from build123d import *

# Parameters (mm, degrees)
SKETCH1_W           = 30
SKETCH1_H           = 41
SKETCH1_R           = 2.25
BOSS_EXTRUDE1_DEPTH = 12
SKETCH3_R           = 3.8
CUT_EXTRUDE2_DEPTH  = 7
FILLET1_R           = 2
SKETCH4_R           = 2.25
CUT_EXTRUDE3_DEPTH  = 53.201532625
CUT_EXTRUDE4_START  = -30
SKETCH5_R           = 3.75
CUT_EXTRUDE4_DEPTH  = 6


with BuildPart() as part:
    # Sketch1 → Boss-Extrude1 (new body)
    with BuildSketch(Plane(origin=(0, 0, 0), x_dir=(1, 0, 0), z_dir=(0, 1, 0))):
        with Locations((-15, 20.5)):
            Rectangle(SKETCH1_W, SKETCH1_H)
        with Locations(Location((-5, 6, 0), (0, 0, 270))):
            Circle(SKETCH1_R, mode=Mode.SUBTRACT)
        with Locations(Location((-5, 26, 0), (0, 0, 270))):
            Circle(SKETCH1_R, mode=Mode.SUBTRACT)
    extrude(amount=BOSS_EXTRUDE1_DEPTH)

    # Sketch3 → Cut-Extrude2 (cut)
    with BuildSketch(Plane(origin=(0, 12, 0), x_dir=(1, 0, 0), z_dir=(0, 1, 0))):
        with Locations(Location((-5, 26, 0), (0, 0, 270))):
            Circle(SKETCH3_R)
        with Locations(Location((-5, 6, 0), (0, 0, 270))):
            Circle(SKETCH3_R)
    extrude(amount=-CUT_EXTRUDE2_DEPTH, mode=Mode.SUBTRACT)

    # Fillet1
    # the kernel refuses this fillet: 2 mm, written as the material it takes off along each edge
    with BuildSketch(Plane(origin=(-28, 10, -2), x_dir=(-1, 0, 0), z_dir=(0, 0, 1))) as fillet1_piece_1_section:
        Polygon((0, 0), (FILLET1_R, 0), (FILLET1_R, -FILLET1_R), (0, -FILLET1_R), align=None)
    fillet1_piece_1 = extrude(amount=FILLET1_R, mode=Mode.PRIVATE)
    fillet1_piece_1 = fillet1_piece_1 - Plane(origin=(-28, 10, -2), x_dir=(0.7071067811865475, -0.7071067811865475, 0), z_dir=(0, 0, 1)) * Sphere(FILLET1_R, mode=Mode.PRIVATE)
    add(fillet1_piece_1, mode=Mode.SUBTRACT)
    with BuildSketch(Plane(origin=(-28, 10, -39), x_dir=(0, 1, 0), z_dir=(-1, 0, 0))) as fillet1_piece_2_section:
        Polygon((0, 0), (FILLET1_R, 0), (FILLET1_R, FILLET1_R), (0, FILLET1_R), align=None)
    fillet1_piece_2 = extrude(amount=FILLET1_R, mode=Mode.PRIVATE)
    fillet1_piece_2 = fillet1_piece_2 - Plane(origin=(-28, 10, -39), x_dir=(0, -0.7071067811865475, 0.7071067811865475), z_dir=(-1, 0, 0)) * Sphere(FILLET1_R, mode=Mode.PRIVATE)
    add(fillet1_piece_2, mode=Mode.SUBTRACT)
    with BuildSketch(Plane(origin=(-2, 10, -2), x_dir=(1, 0, 0), z_dir=(0, 0, 1))) as fillet1_piece_3_section:
        Polygon((0, 0), (FILLET1_R, 0), (FILLET1_R, FILLET1_R), (0, FILLET1_R), align=None)
    fillet1_piece_3 = extrude(amount=FILLET1_R, mode=Mode.PRIVATE)
    fillet1_piece_3 = fillet1_piece_3 - Plane(origin=(-2, 10, -2), x_dir=(-0.7071067811865475, -0.7071067811865475, 0), z_dir=(0, 0, 1)) * Sphere(FILLET1_R, mode=Mode.PRIVATE)
    add(fillet1_piece_3, mode=Mode.SUBTRACT)
    with BuildSketch(Plane(origin=(-2, 10, -39), x_dir=(0, 1, 0), z_dir=(1, 0, 0))) as fillet1_piece_4_section:
        Polygon((0, 0), (FILLET1_R, 0), (FILLET1_R, -FILLET1_R), (0, -FILLET1_R), align=None)
    fillet1_piece_4 = extrude(amount=FILLET1_R, mode=Mode.PRIVATE)
    fillet1_piece_4 = fillet1_piece_4 - Plane(origin=(-2, 10, -39), x_dir=(0, -0.7071067811865475, 0.7071067811865475), z_dir=(1, 0, 0)) * Sphere(FILLET1_R, mode=Mode.PRIVATE)
    add(fillet1_piece_4, mode=Mode.SUBTRACT)
    with BuildSketch(Plane(origin=(-2, 2, -2), x_dir=(1, 0, 0), z_dir=(0, 0, 1))) as fillet1_piece_5_section:
        Polygon((0, 0), (FILLET1_R, 0), (FILLET1_R, -FILLET1_R), (0, -FILLET1_R), align=None)
    fillet1_piece_5 = extrude(amount=FILLET1_R, mode=Mode.PRIVATE)
    fillet1_piece_5 = fillet1_piece_5 - Plane(origin=(-2, 2, -2), x_dir=(-0.7071067811865475, 0.7071067811865475, 0), z_dir=(0, 0, 1)) * Sphere(FILLET1_R, mode=Mode.PRIVATE)
    add(fillet1_piece_5, mode=Mode.SUBTRACT)
    with BuildSketch(Plane(origin=(-28, 2, -2), x_dir=(-1, 0, 0), z_dir=(0, 0, 1))) as fillet1_piece_6_section:
        Polygon((0, 0), (FILLET1_R, 0), (FILLET1_R, FILLET1_R), (0, FILLET1_R), align=None)
    fillet1_piece_6 = extrude(amount=FILLET1_R, mode=Mode.PRIVATE)
    fillet1_piece_6 = fillet1_piece_6 - Plane(origin=(-28, 2, -2), x_dir=(0.7071067811865475, 0.7071067811865475, 0), z_dir=(0, 0, 1)) * Sphere(FILLET1_R, mode=Mode.PRIVATE)
    add(fillet1_piece_6, mode=Mode.SUBTRACT)
    with BuildSketch(Plane(origin=(-28, 2, -39), x_dir=(0, -1, 0), z_dir=(-1, 0, 0))) as fillet1_piece_7_section:
        Polygon((0, 0), (FILLET1_R, 0), (FILLET1_R, -FILLET1_R), (0, -FILLET1_R), align=None)
    fillet1_piece_7 = extrude(amount=FILLET1_R, mode=Mode.PRIVATE)
    fillet1_piece_7 = fillet1_piece_7 - Plane(origin=(-28, 2, -39), x_dir=(0, 0.7071067811865475, 0.7071067811865475), z_dir=(-1, 0, 0)) * Sphere(FILLET1_R, mode=Mode.PRIVATE)
    add(fillet1_piece_7, mode=Mode.SUBTRACT)
    with BuildSketch(Plane(origin=(-2, 2, -39), x_dir=(0, -1, 0), z_dir=(1, 0, 0))) as fillet1_piece_8_section:
        Polygon((0, 0), (FILLET1_R, 0), (FILLET1_R, FILLET1_R), (0, FILLET1_R), align=None)
    fillet1_piece_8 = extrude(amount=FILLET1_R, mode=Mode.PRIVATE)
    fillet1_piece_8 = fillet1_piece_8 - Plane(origin=(-2, 2, -39), x_dir=(0, 0.7071067811865475, 0.7071067811865475), z_dir=(1, 0, 0)) * Sphere(FILLET1_R, mode=Mode.PRIVATE)
    add(fillet1_piece_8, mode=Mode.SUBTRACT)
    with BuildSketch(Plane(origin=(-30, 12, -2), x_dir=(0, -1, 0), z_dir=(0, 0, -1)), Plane(origin=(0, 12, -39), x_dir=(0, -1, 0), z_dir=(0, 0, 1))) as fillet1_piece_9:
        with BuildLine():
            CenterArc((FILLET1_R, -FILLET1_R), FILLET1_R, 90, 90)
            Line((0, -FILLET1_R), (0, 0))
            Line((0, 0), (FILLET1_R, 0))
        make_face()
    extrude(amount=37, mode=Mode.SUBTRACT)
    with BuildSketch(Plane(origin=(-2, 12, 0), x_dir=(0, -1, 0), z_dir=(-1, 0, 0)), Plane(origin=(-28, 0, -41), x_dir=(0, 0, 1), z_dir=(1, 0, 0))) as fillet1_piece_10:
        with BuildLine():
            CenterArc((FILLET1_R, -FILLET1_R), FILLET1_R, 90, 90)
            Line((0, -FILLET1_R), (0, 0))
            Line((0, 0), (FILLET1_R, 0))
        make_face()
    extrude(amount=26, mode=Mode.SUBTRACT)
    with BuildSketch(Plane(origin=(-2, 0, 0), x_dir=(0, 1, 0), z_dir=(-1, 0, 0)), Plane(origin=(-28, 12, -41), x_dir=(0, 0, 1), z_dir=(1, 0, 0))) as fillet1_piece_11:
        with BuildLine():
            CenterArc((FILLET1_R, FILLET1_R), FILLET1_R, 180, 90)
            Line((0, FILLET1_R), (0, 0))
            Line((0, 0), (FILLET1_R, 0))
        make_face()
    extrude(amount=26, mode=Mode.SUBTRACT)
    with BuildSketch(Plane(origin=(-30, 0, -2), x_dir=(0, 1, 0), z_dir=(0, 0, -1)), Plane(origin=(0, 0, -39), x_dir=(0, 1, 0), z_dir=(0, 0, 1))) as fillet1_piece_12:
        with BuildLine():
            CenterArc((FILLET1_R, FILLET1_R), FILLET1_R, 180, 90)
            Line((0, FILLET1_R), (0, 0))
            Line((0, 0), (FILLET1_R, 0))
        make_face()
    extrude(amount=37, mode=Mode.SUBTRACT)
    with BuildSketch(Plane(origin=(0, 2, 0), x_dir=(-1, 0, 0), z_dir=(0, 1, 0)), Plane(origin=(0, 2, -41), x_dir=(0, 0, 1), z_dir=(0, 1, 0))) as fillet1_piece_13:
        with BuildLine():
            CenterArc((FILLET1_R, -FILLET1_R), FILLET1_R, 90, 90)
            Line((0, -FILLET1_R), (0, 0))
            Line((0, 0), (FILLET1_R, 0))
        make_face()
    extrude(amount=8, mode=Mode.SUBTRACT)
    with BuildSketch(Plane(origin=(-30, 2, 0), x_dir=(1, 0, 0), z_dir=(0, 1, 0)), Plane(origin=(-30, 2, -41), x_dir=(0, 0, 1), z_dir=(0, 1, 0))) as fillet1_piece_14:
        with BuildLine():
            CenterArc((FILLET1_R, FILLET1_R), FILLET1_R, 180, 90)
            Line((0, FILLET1_R), (0, 0))
            Line((0, 0), (FILLET1_R, 0))
        make_face()
    extrude(amount=8, mode=Mode.SUBTRACT)

    # Sketch4 → Cut-Extrude3 (cut, through all)
    with BuildSketch(Plane.ZY.offset(30)):
        with Locations((-34, 5.5)):
            Circle(SKETCH4_R)
        with Locations((-18, 5.5)):
            Circle(SKETCH4_R)
    extrude(amount=-CUT_EXTRUDE3_DEPTH, mode=Mode.SUBTRACT)

    # Sketch5 → Cut-Extrude4 (cut)
    with BuildSketch(Plane.ZY.offset(30).offset(CUT_EXTRUDE4_START)):
        with Locations(Location((-34, 5.5, 0), (0, 0, 248.960530219))):
            Circle(SKETCH5_R)
        with Locations(Location((-18, 5.5, 0), (0, 0, 248.960530219))):
            Circle(SKETCH5_R)
    extrude(amount=CUT_EXTRUDE4_DEPTH, mode=Mode.SUBTRACT)


solid = part.part
Check sheet for the modelled part. Datum: model origin and axes. Units: mm. A direction names the side the tool comes from. Round coordinates to 2 decimals unless told otherwise and drop trailing zeros. Write each loop counter-clockwise with the first axis right and the second up, starting at its lowest first coordinate (ties: lowest second). Pieces come first, ordered by that corner, then holes. Notation, with made-up numbers: (36, 62.25) -> (90, 62.25) arc R30 ccw to (90, 90.25) -> close; hole circle Ø7 at (40.5, 28). An arc over 180 degrees is marked (long way). Answer as CSV lines item,"result". Start each with the question number.
1) Tool access check on faces 5 (the cylindrical face through (-0.57, 11.4, -20.76)), 6 (the cylindrical face through (-6.46, 8.55, -2.49)), 7 (the cylindrical face through (-2.958, 1.757, -18.233)). Record the directions out of +Z, -Z, +X, -X, +Y, -Y that give a thin tool (end or side, any length) a straight path to the whole face; none if there is none.
2) Section check B-B on x = -5.5. Enter the section's corners in (y, z).
3) Go/stop test with flat-tipped pins: P1, Ø4, axis at y = 5.5, z = -33.5, coming from the +X side; P2, Ø1, axis at x = -7, z = -10, coming from the -Y side; P3, Ø7, axis at x = -5, z = -6, coming from the +Y side; P4, Ø3.5, axis at y = 5.5, z = -18, coming from the -X side. Record where each tip stops, or that it passes through.
4) Section check A-A on y = 5.5. Enter the section's corners in (x, z).
5) Section check D-D on z = -34. Enter the section's corners in (x, y), and give its area (3 significant figures).
6) Release check for a two-part mould opening along Y. For faces 1 (the flat face through (-6, 6.4, -36.3)), 2 (the flat face through (-15, 0, -21)), 3 (the cylindrical face through (-14.82, 11.4, -0.57)), 4 (the cylindrical face through (-0.6, 5.94, -0.57)) record: pulls with the +Y half, pulls with the -Y half, needs draft (parallel to the pull), parting line crosses it, or undercut.
7) Material ranges on line 1 (X direction, y = 8.5, z = -26); line 2 (Z direction, x = -5, y = 10.25); line 3 (Z direction, x = -3, y = 8.75), recorded low to high. Write a range as from..to.
8) Section check C-C on y = 8.5. Enter the section's corners in (x, z).
Found:
1,face 5,"+Z, -Z, +X, +Y"
1,face 6,"+Y"
1,face 7,"+X"
2,outline,"(0, -39) arc R2 ccw to (2, -41) -> (10, -41) arc R2 ccw to (12, -39) -> (12, -29.77) -> (5, -29.77) -> (5, -28.19) -> (0, -28.19) -> close; (0, -23.81) -> (5, -23.81) -> (5, -22.23) -> (12, -22.23) -> (12, -9.77) -> (5, -9.77) -> (5, -8.19) -> (0, -8.19) -> close; (0, -3.81) -> (5, -3.81) -> (5, -2.23) -> (12, -2.23) -> (12, -2) arc R2 ccw to (10, 0) -> (2, 0) arc R2 ccw to (0, -2) -> close; hole circle Ø7.5 at (5.5, -34); hole circle Ø7.5 at (5.5, -18)"
3,P1,"stops at x = -6"
3,P2,"stops at y = 0"
3,P3,"stops at y = 5"
3,P4,"passes through"
4,outline,"(-30, -39) arc R2 ccw to (-28, -41) -> (-2, -41) arc R2 ccw to (0, -39) -> (0, -37.75) -> (-6, -37.75) -> (-6, -36.25) -> (-30, -36.25) -> close; (-30, -31.75) -> (-6, -31.75) -> (-6, -30.25) -> (0, -30.25) -> (0, -21.75) -> (-6, -21.75) -> (-6, -20.25) -> (-30, -20.25) -> close; (-30, -15.75) -> (-6, -15.75) -> (-6, -14.25) -> (0, -14.25) -> (0, -2) arc R2 ccw to (-2, 0) -> (-28, 0) arc R2 ccw to (-30, -2) -> close; hole circle Ø7.6 at (-5, -26); hole circle Ø7.6 at (-5, -6)"
5,outline,"(-30, 2) arc R2 ccw to (-28, 0) -> (-2, 0) arc R2 ccw to (-0.02, 1.75) -> (-6, 1.75) -> (-6, 3.25) -> (-30, 3.25) -> close; (-30, 7.75) -> (-6, 7.75) -> (-6, 9.25) -> (0, 9.25) -> (0, 10) arc R2 ccw to (-2, 12) -> (-28, 12) arc R2 ccw to (-30, 10) -> close"
5,area,"204 mm^2"
6,face 1,"undercut"
6,face 2,"pulls with the -Y half"
6,face 3,"pulls with the +Y half"
6,face 4,"needs draft"
7,line 1,"x = -30..-8.8, -1.2..0"
7,line 2,"z = -40.98..-29.8, -22.2..-9.8, -2.2..-0.02"
7,line 3,"z = -41..-35.87, -32.13..-29.23, -22.77..-19.87, -16.13..-9.23, -2.77..0"
8,outline,"(-30, -39) arc R2 ccw to (-28, -41) -> (-2, -41) arc R2 ccw to (0, -39) -> (0, -36.25) -> (-6, -36.25) -> (-6, -31.75) -> (0, -31.75) -> (0, -20.25) -> (-6, -20.25) -> (-6, -15.75) -> (0, -15.75) -> (0, -2) arc R2 ccw to (-2, 0) -> (-28, 0) arc R2 ccw to (-30, -2) -> close; hole circle Ø7.6 at (-5, -26); hole circle Ø7.6 at (-5, -6)"
